Geometry check sheet. Reference: the model listing, model coordinates, mm. A direction names the side the tool comes from. Give positions to 0.01 mm unless a question says otherwise; leave off trailing zeros. Order: outer loops, then holes, each group sorted by start corner. A loop starts at its lowest first (then second) coordinate and runs counter-clockwise, first axis right, second up.
from build123d import *

# Parameters (mm, degrees)
F0_W      = 110
F0_H      = 126
F1_DEPTH  = 6.5
F2_W      = 110
F2_H      = 6.5
F3_DEPTH  = 38.1
F4_R      = 1.8
F5_DEPTH  = 14.3
F6_R      = 18
F7_R      = 18
F8_W      = 6.5
F8_H      = 146.1
F9_DEPTH  = 20.8
F10_W     = 38.1
F10_H     = 20.8
F11_DEPTH = 133.7
F13_R     = 3


# Not quite as in the source:
# - a feature of the source that left no trace in its solid (it failed there, or was rolled back) is left out


with BuildPart() as f1:
    # F0 (on Top) → F1 (new body)
    with BuildSketch(Plane.XY):
        with Locations((55, -63)):
            Rectangle(F0_W, F0_H)
    extrude(amount=F1_DEPTH)

    # F2 (on face) → F3 (join)
    with BuildSketch(Plane(origin=(0, 0, 0), x_dir=(-1, 0, 0), z_dir=(0, 1, 0))):
        with Locations((-55, 3.25)):
            Rectangle(F2_W, F2_H)
    extrude(amount=F3_DEPTH)

    # F4 (on face) → F5 (cut)
    with BuildSketch(Plane.XY.offset(6.5)):
        with Locations((55, 28.0327554792)):
            Circle(F4_R)
    extrude(amount=-F5_DEPTH, mode=Mode.SUBTRACT)

    # F6
    f6_edges = [f1.edges().sort_by_distance(p)[0] for p in [
        (110, -126, 3.25),
    ]]
    fillet(f6_edges, radius=F6_R)

    # F7
    f7_edges = [f1.edges().sort_by_distance(p)[0] for p in [
        (0, -126, 3.25),
    ]]
    fillet(f7_edges, radius=F7_R)

    # F8 (on face) → F9 (join)
    with BuildSketch(Plane(origin=(0, 0, 0), x_dir=(1, 0, 0), z_dir=(0, 0, -1))):
        with Locations((3.25, 34.95)):
            Rectangle(F8_W, F8_H)
        with Locations((106.75, 34.95)):
            Rectangle(F8_W, F8_H)
    extrude(amount=F9_DEPTH)

    # F10 (on face) → F11 (cut)
    with BuildSketch(Plane.YZ.offset(110)):
        with Locations((19.05, -10.4)):
            Rectangle(F10_W, F10_H)
        Polygon((0, -20.8), (-108, 0), (-108, -20.8), align=None)
    extrude(amount=-F11_DEPTH, mode=Mode.SUBTRACT)

    # F13
    f13_edges = [f1.edges().sort_by_distance(p)[0] for p in [
        (106.75, 0, -20.8),
        (3.25, 0, -20.8),
    ]]
    fillet(f13_edges, radius=F13_R)


solid = f1.part
Item 1: Sectioned sample at A-A (x = 55). Enter the section's corners in (y, z), and give its area (3 significant figures).
Reported:
outline: (-126, 0) - (26.23, 0) - (26.23, 6.5) - (-126, 6.5) - close; (29.83, 0) - (38.1, 0) - (38.1, 6.5) - (29.83, 6.5) - close
area: 1,040 mm2
Item 2: Gauge pin test, flat ends, axial feed: pin 1 (7 mm diameter, centred on x = 108.5, z = -10.5, fed in from +Y); pin 2 (3 mm diameter, centred on x = 66, y = -97.5, fed in from -Z); pin 3 (3 mm diameter, centred on x = 94, z = 2.5, fed in from -Y). Record the tip position at first contact, or that the pin passes through.
Reported:
pin 1: stops at y = 0
pin 2: stops at z = 0
pin 3: stops at y = -125.99
Item 3: Sectioned sample at C-C (x = 69.5). Enter the section's corners in (y, z), and give its area (3 significant figures).
Reported:
outline: (-126, 0) - (38.1, 0) - (38.1, 6.5) - (-126, 6.5) - close
area: 1,070 mm2
Item 4: Set-up check for faces 1 (the flat face through (103.5, -41, -8)), 2 (the flat face through (106.796, -55.053, -10.197)), 3 (the flat face through (3, 0, -9)): record each of +Z, -Z, +X, -X, +Y, -Y from which the full face is reachable in a straight line by a thin tool's end or side.
Reported:
face 1: -Z, +Y, -Y
face 2: -Z, +X, -X, -Y
face 3: -Z, +X, -X, +Y
Item 5: Draft check along X on faces 4 (the flat face through (107, 0, -9)), 5 (the cylindrical face through (104.867, -120.587, 3.296)), 6 (the cylindrical face through (55.831, 26.436, 3.296)). Enter one of: released by +X, released by -X, zero draft, split by the parting line, or undercut.
Reported:
face 4: zero draft
face 5: released by +X
face 6: undercut
Item 6: Sectioned sample at D-D (y = -96). Enter the section's corners in (x, z), and give its area (3 significant figures).
Reported:
outline: (0, -2.31) - (6.5, -2.31) - (6.5, 0) - (103.5, 0) - (103.5, -2.31) - (110, -2.31) - (110, 6.5) - (0, 6.5) - close
area: 745 mm2
Item 7: Scan lines: L1, parallel to X at y = -57.5, z = -9.5; L2, parallel to Y at x = 55, z = 3.5; L3, parallel to Z at x = 91.5, y = -16. Record each from-to range of solid material in increasing order.
Reported:
L1: x = 0 to 6.5, 103.5 to 110
L2: y = -126 to 26.23, 29.83 to 38.1
L3: z = 0 to 6.5
Item 8: Sectioned sample at B-B (z = -9). Enter the section's corners in (x, y), and give its area (4 significant figures).
Reported:
outline: (0, -61.27) - (6.5, -61.27) - (6.5, 0) - (0, 0) - close; (103.5, -61.27) - (110, -61.27) - (110, 0) - (103.5, 0) - close
area: 796.5 mm2
